Geometry check sheet. Reference: the model listing, model coordinates, mm. Round coordinates to 2 decimals unless told otherwise and drop trailing zeros. Loops run counter-clockwise (first coordinate to the right, second up) from the corner with the lowest first, then second, coordinate; pieces in that order, holes last. Notation, with made-up numbers: M 50,64 L 63,64 A20 cw 63,102 Z; hole C 61.25,-33 d2. An arc over 180 degrees is marked long. Use one line per item in the form item = value. Start each with the question number.
1. Cross-section at A-A (y = 0). Record the boundary of the cut face in (x, z), then the cut area to 3 significant figures.
2. Cross-section at B-B (z = -50.5). Record the boundary of the cut face in (x, y), then the cut area to 3 significant figures.
3. Material ranges on line 1 (Z direction, x = 855, y = -3); line 2 (Z direction, x = 691.5, y = 48); line 3 (Y direction, x = 66, z = -5.5), recorded low to high.
4. Cross-section at C-C (x = 525.5). Record the boundary of the cut face in (y, z).
5. Go/stop test with flat-tipped pins: pin 1 (3.5 mm diameter, centred on x = 165, z = -2.06, fed in from -Y); pin 2 (6 mm diameter, centred on x = 772, y = -45, fed in from -Z); pin 3 (8 mm diameter, centred on x = 372, y = 32.5, fed in from +Z). Record where each tip stops, or that it passes through.
6. Draft check along Z on faces 1 (the flat face through (0, -62, 40)), 2 (the cylindrical face through (456.3, 74.388, -16.519)), 3 (the cylindrical face through (456.3, 71.86, -15.96)). Enter one of: pulls with the +Z half, pulls with the -Z half, needs draft (parallel to the pull), parting line crosses it, or undercut.
```python
from build123d import *

# Parameters (mm, degrees)
ESQUISSE1_W          = 900
ESQUISSE1_H          = 2.5908
D_GAGEMENT_M51_D     = 5.5
D_GAGEMENT_M51_DEPTH = 10
D_GAGEMENT_M51_TIP   = 1.652366702


with BuildPart() as part:
    # Esquisse1 → Révolution1 (revolve)
    with BuildSketch(Plane.XY, mode=Mode.PRIVATE) as r_volution1_sk:
        with Locations((450, 74.9046)):
            Rectangle(ESQUISSE1_W, ESQUISSE1_H)
    revolve(r_volution1_sk.sketch.rotate(Axis((0, 0, 0), (1, 0, 0)), 90), axis=Axis((0, 0, 0), (1, 0, 0)))

    # Dégagement M51
    with Locations(Plane(origin=(0, 76.2, 0), x_dir=(1, 0, 0), z_dir=(0, 1, 0))):
        with Locations((165, 2.06190404), (87.5, 2.06190404), (10, 2.06190404)):
            Hole(D_GAGEMENT_M51_D / 2, depth=D_GAGEMENT_M51_DEPTH)
            with Locations((0, 0, -(D_GAGEMENT_M51_DEPTH + D_GAGEMENT_M51_TIP / 2))):  # 118° drill point
                Cone(0, D_GAGEMENT_M51_D / 2, D_GAGEMENT_M51_TIP, mode=Mode.SUBTRACT)


solid = part.part
```
Reported:
q1.outline = M 0,-76.2 L 900,-76.2 L 900,-73.61 L 0,-73.61 Z; M 0,73.61 L 900,73.61 L 900,76.2 L 0,76.2 Z
q1.area = 4,660 mm²
q2.outline = M 0,-57.06 L 900,-57.06 L 900,-53.55 L 0,-53.55 Z; M 0,53.55 L 900,53.55 L 900,57.06 L 0,57.06 Z
q2.area = 6,320 mm²
q3.line_1 = -76.14 to -73.55, 73.55 to 76.14
q3.line_2 = -59.18 to -55.81, 55.81 to 59.18
q3.line_3 = -76 to -73.4, 73.4 to 76
q4.outline = C 0,0 d152.4; hole C 0,0 d147.22
q5.pin_1 = -76.2
q5.pin_2 = -63.58
q5.pin_3 = 70.67
q6.face_1 = needs draft
q6.face_2 = parting line crosses it
q6.face_3 = undercut
